Model file for the job. Use its own axes, mm. A direction names the side the tool comes from. Coordinates: 2 decimals unless noted, no trailing zeros. Write each loop counter-clockwise with the first axis right and the second up, starting at its lowest first coordinate (ties: lowest second). Pieces come first, ordered by that corner, then holes. Notation, with made-up numbers: M 83.5,14.5 L 135.5,14.5 A35 cw 135.5,53.5 Z; hole C -2.5,-13 d3. An arc over 180 degrees is marked long. Use CSV: the item, a comma, the result in double quotes. Start each with the question number.
from build123d import *

# Parameters (mm, degrees)
SKETCH4_W               = 2449.5
SKETCH4_H               = 930
SKETCH4_W_2             = 2149.5
SKETCH4_H_2             = 530
BOSS_EXTRUDE2_DEPTH     = 30
SKETCH6_W               = 2449.5
SKETCH6_H               = 930
SKETCH6_W_2             = 2349.5
SKETCH6_H_2             = 830
BOSS_EXTRUDE3_DEPTH     = 100
SKETCH8_W               = 174.417097876
SKETCH8_H               = 150
BOSS_EXTRUDE4_DEPTH     = 175
CUT_EXTRUDE1_DEPTH      = 680
CUT_EXTRUDE1_DEPTH_BACK = 150
SKETCH10_R              = 30
FILLET1_R               = 80


with BuildPart() as part:
    # Sketch4 → Boss-Extrude2 (new body)
    with BuildSketch(Plane(origin=(0, 0, 0), x_dir=(1, 0, 0), z_dir=(0, 1, 0))):
        with Locations((2350.564429087, 865.22075714)):
            Rectangle(SKETCH4_W, SKETCH4_H)
        with Locations((2350.564429087, 865.22075714)):
            Rectangle(SKETCH4_W_2, SKETCH4_H_2, mode=Mode.SUBTRACT)
    extrude(amount=BOSS_EXTRUDE2_DEPTH)

    # Sketch6 → Boss-Extrude3 (add)
    with BuildSketch(Plane(origin=(0, 30, 0), x_dir=(1, 0, 0), z_dir=(0, 1, 0))):
        with Locations((2350.564429087, 865.22075714)):
            Rectangle(SKETCH6_W, SKETCH6_H)
        with Locations((2350.564429087, 865.22075714)):
            Rectangle(SKETCH6_W_2, SKETCH6_H_2, mode=Mode.SUBTRACT)
    extrude(amount=BOSS_EXTRUDE3_DEPTH)

    # Sketch8 → Boss-Extrude4 (add)
    with BuildSketch(Plane(origin=(0, 30, 0), x_dir=(1, 0, 0), z_dir=(0, 1, 0))):
        with Locations((1546.094821657, 1205.22075714)):
            Rectangle(SKETCH8_W, SKETCH8_H)
        with Locations((1546.094821657, 525.22075714)):
            Rectangle(SKETCH8_W, SKETCH8_H)
    extrude(amount=BOSS_EXTRUDE4_DEPTH)

    # Sketch10 → Cut-Extrude1 (cut, two sides: drawn at the far end of the back side and taken through both)
    with BuildSketch(Plane.XY.offset(-1130.22075714).offset(-CUT_EXTRUDE1_DEPTH_BACK)):
        with Locations(Location((1544.625999864, 116.419579706, 0), (0, 0, 180))):
            Circle(SKETCH10_R)
    extrude(amount=CUT_EXTRUDE1_DEPTH + CUT_EXTRUDE1_DEPTH_BACK, mode=Mode.SUBTRACT)

    # Fillet1
    # the kernel refuses this fillet: 80 mm, written as the material it takes off along each edge
    with BuildSketch(Plane(origin=(1633.303370595, 205, -1280.22075714), x_dir=(0, -1, 0), z_dir=(0, 0, 1)), Plane(origin=(1458.886272719, 205, -450.22075714), x_dir=(0, -1, 0), z_dir=(0, 0, -1))) as fillet1_piece_1:
        with BuildLine():
            CenterArc((FILLET1_R, -FILLET1_R), FILLET1_R, 90, 90)
            Line((0, -FILLET1_R), (0, 0))
            Line((0, 0), (FILLET1_R, 0))
        make_face()
    extrude(amount=350, mode=Mode.SUBTRACT)
    with BuildSketch(Plane(origin=(1458.886272719, 205, -930.22075714), x_dir=(1, 0, 0), z_dir=(0, 0, -1)), Plane(origin=(1633.303370595, 205, -800.22075714), x_dir=(-1, 0, 0), z_dir=(0, 0, 1))) as fillet1_piece_2:
        with BuildLine():
            CenterArc((FILLET1_R, FILLET1_R), FILLET1_R, 180, 90)
            Line((0, FILLET1_R), (0, 0))
            Line((0, 0), (FILLET1_R, 0))
        make_face()
    extrude(amount=350, mode=Mode.SUBTRACT)


solid = part.part
1) Band-saw the part on B-B on y = 52. List the corners of the cut face in (x, z), then the cut area to 3 significant figures.
2) Wall check: L1, parallel to X at y = 36.5, z = -1265.5; L2, parallel to Z at x = 2185.5, y = 29.5; L3, parallel to Z at x = 3307, y = 36.5. Give the ranges that are in metal, low to high. Write a range as [from, to].
3) Band-saw the part on C-C on z = -694. List the corners of the cut face in (x, y).
4) Two-plate mould, pull along Z, no slides. Class faces 1 (the face through (1982, 130, -1281)), 2 (the face through (1458.886, 77, -524)), 3 (the face through (1545, 167, -1280.221)): pulls with the +Z half, pulls with the -Z half, needs draft (parallel to the pull), parting line crosses it, or undercut.
5) Band-saw the part on D-D on z = -479. List the corners of the cut face in (x, y), then the cut area to 3 significant figures.
6) Tool access for faces 4 (the face through (2107, 26, -1130.221)), 5 (the face through (2333, 64, -400.221)), 6 (the face through (1175.814, 79, -859)), 7 (the face through (1545, 113, -1280.221)): list every direction of +Z, -Z, +X, -X, +Y, -Y with a clear straight run to the whole face (end or side of a thin tool).
7) Band-saw the part on A-A on x = 2018.5. List the corners of the cut face in (y, z), then the cut area to 3 significant figures.
Findings below:
1,outline,"M 1125.81,-1330.22 L 3575.31,-1330.22 L 3575.31,-400.22 L 1125.81,-400.22 Z; hole M 1175.81,-1280.22 L 1458.89,-1280.22 L 1458.89,-1130.22 L 1633.3,-1130.22 L 1633.3,-1280.22 L 3525.31,-1280.22 L 3525.31,-450.22 L 1633.3,-450.22 L 1633.3,-600.22 L 1458.89,-600.22 L 1458.89,-450.22 L 1175.81,-450.22 Z"
1,area,"380,000 mm2"
2,L1,"x = [1125.81, 1175.81], [1458.89, 1633.3], [3525.31, 3575.31]"
2,L2,"z = [-1330.22, -1130.22], [-600.22, -400.22]"
2,L3,"z = [-1330.22, -1280.22], [-450.22, -400.22]"
3,outline,"M 1125.81,0 L 1275.81,0 L 1275.81,30 L 1175.81,30 L 1175.81,130 L 1125.81,130 Z; M 3425.31,0 L 3575.31,0 L 3575.31,130 L 3525.31,130 L 3525.31,30 L 3425.31,30 Z"
4,face 1,"needs draft"
4,face 2,"undercut"
4,face 3,"pulls with the -Z half"
5,outline,"M 1125.81,0 L 3575.31,0 L 3575.31,130 L 3525.31,130 L 3525.31,30 L 1633.3,30 L 1633.3,125 A80 ccw 1553.3,205 L 1538.89,205 A80 ccw 1458.89,125 L 1458.89,30 L 1175.81,30 L 1175.81,130 L 1125.81,130 Z; hole C 1544.63,116.42 d60"
5,area,"108,000 mm2"
6,face 4,"+Y, -Y"
6,face 5,"+Z, +X, -X, +Y, -Y"
6,face 6,"+Y"
6,face 7,"none"
7,outline,"M 0,-1330.22 L 130,-1330.22 L 130,-1280.22 L 30,-1280.22 L 30,-1130.22 L 0,-1130.22 Z; M 0,-600.22 L 30,-600.22 L 30,-450.22 L 130,-450.22 L 130,-400.22 L 0,-400.22 Z"
7,area,"22,000 mm2"
